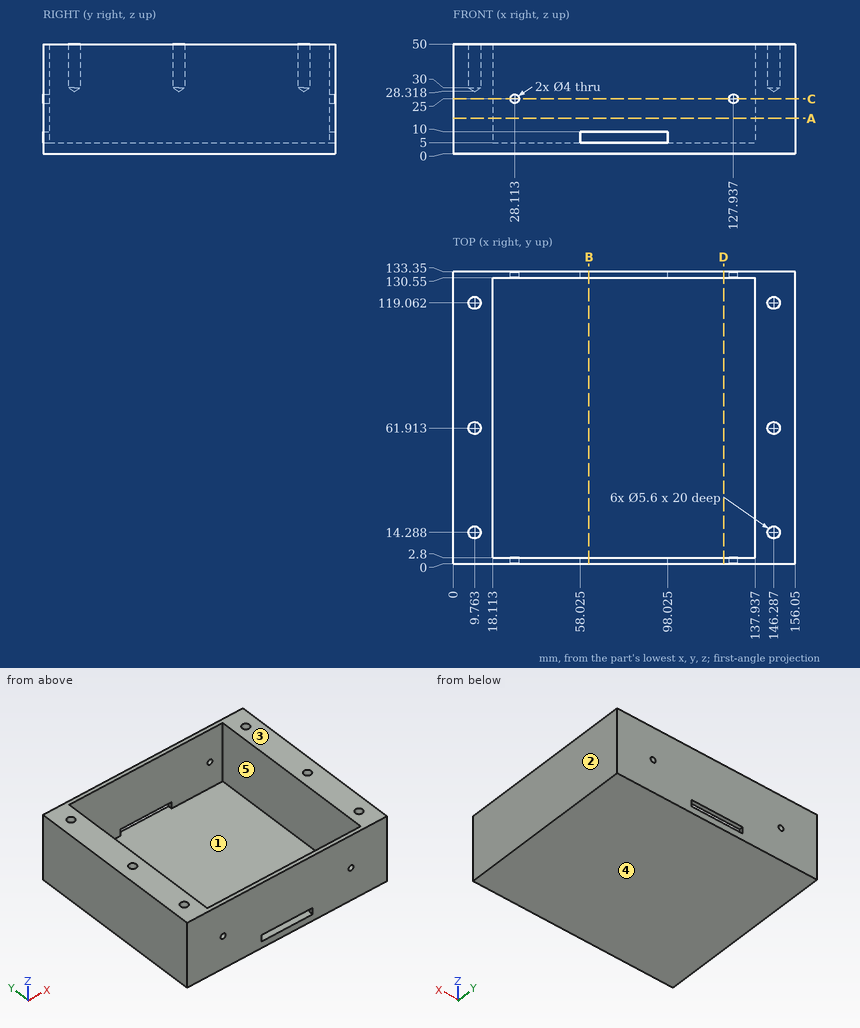
Geometry: see drawing. Coordinates: mm, zero at the bounding-box minimum. A direction names the side the tool comes from. Coordinates: 2 decimals unless noted, no trailing zeros. Order: outer loops, then holes, each group sorted by start corner. A loop starts at its lowest first (then second) coordinate and runs counter-clockwise, first axis right, second up. Notation, with made-up numbers: (27, -6.75) -> (52, -6.75) arc R27 ccw to (52, 20.25) -> close; hole circle Ø2 at (20, -21). An arc over 180 degrees is marked (long way). Write each question's results on one line, items separated by ' | '. Start each with the question number.
1) Mould query, pull axis X, two halves, no side actions, for the marked faces 1, 2 and 3. Classes: released by +X, released by -X, zero draft, split by the parting line, or undercut.
2) First-contact query: pin 1 (3 mm diameter, centred on y = 32.5, z = 39.5, fed in from -X); pin 2 (4.5 mm diameter, centred on x = 9.763, y = 119.062, fed in from +Z). Flat tips, straight axial feed; report the tip coordinate or a pass-through.
3) Cut plane A-A, the plane z = 16. Output: boundary loops of the cut face in (x, y), and give its area (3 significant figures).
4) Set-up query: the marked faces 4 and 5. Return all of +Z, -Z, +X, -X, +Y, -Y with unobstructed straight access to the full face (end or side cutting, diameter ignored); none if empty.
5) Cut plane C-C, the plane z = 25. Output: boundary loops of the cut face in (x, y).
6) Cut plane B-B, the plane x = 62. Output: boundary loops of the cut face in (y, z).
7) Material intervals for line 1 along X through (y, z) = (81.5, 47); line 2 along Y through (x, z) = (31, 15.5); line 3 along Z through (x, y) = (34, 105.5), sorted ascending.
8) Cut plane D-D, the plane x = 123.5. Output: boundary loops of the cut face in (y, z).
Checks:
1) face 1: undercut | face 2: released by +X | face 3: zero draft
2) pin 1: x = 0 | pin 2: z = 29.67
3) outline: (0, 0) -> (156.05, 0) -> (156.05, 133.35) -> (0, 133.35) -> close; hole (18.11, 2.8) -> (137.94, 2.8) -> (137.94, 130.55) -> (18.11, 130.55) -> close | area: 5,500 mm^2
4) face 4: -Z, +X, -X, +Y, -Y | face 5: +Z
5) outline: (0, 0) -> (26.11, 0) -> (26.11, 2.8) -> (18.11, 2.8) -> (18.11, 130.55) -> (26.11, 130.55) -> (26.11, 133.35) -> (0, 133.35) -> close; (30.11, 0) -> (125.94, 0) -> (125.94, 2.8) -> (30.11, 2.8) -> close; (30.11, 130.55) -> (125.94, 130.55) -> (125.94, 133.35) -> (30.11, 133.35) -> close; (129.94, 0) -> (156.05, 0) -> (156.05, 133.35) -> (129.94, 133.35) -> (129.94, 130.55) -> (137.94, 130.55) -> (137.94, 2.8) -> (129.94, 2.8) -> close
6) outline: (0, 0) -> (133.35, 0) -> (133.35, 5) -> (0, 5) -> close; (0, 10) -> (2.8, 10) -> (2.8, 50) -> (0, 50) -> close; (130.55, 10) -> (133.35, 10) -> (133.35, 50) -> (130.55, 50) -> close
7) line 1: 0 to 18.11, 137.94 to 156.05 | line 2: 0 to 2.8, 130.55 to 133.35 | line 3: 0 to 5
8) outline: (0, 0) -> (133.35, 0) -> (133.35, 50) -> (130.55, 50) -> (130.55, 5) -> (2.8, 5) -> (2.8, 50) -> (0, 50) -> close
